from build123d import *

# Parameters (mm, degrees)
BOSS_EXTRUDE1_DEPTH = 11
SKETCH3_W           = 22
SKETCH3_H           = 3
BOSS_EXTRUDE2_DEPTH = 14
BOSS_EXTRUDE3_DEPTH = 5
SKETCH5_R           = 1.75
CUT_EXTRUDE1_DEPTH  = 36.096650541
SKETCH6_W           = 9
SKETCH6_H           = 9
BOSS_EXTRUDE4_DEPTH = 5
SKETCH10_R          = 2.25
CUT_EXTRUDE2_DEPTH  = 34.584744739
FILLET1_R           = 0.75
FILLET2_SIZE        = 10
SKETCH12_W          = 9
SKETCH12_H          = 32.0178
BOSS_EXTRUDE5_DEPTH = 62
CUT_EXTRUDE4_DEPTH  = 9
SKETCH14_R          = 2.5
CUT_EXTRUDE5_DEPTH  = 9.75
SKETCH15_R          = 1.7
CUT_EXTRUDE6_DEPTH  = 5
SKETCH16_R          = 2.5
CUT_EXTRUDE7_DEPTH  = 1.6
FILLET3_R           = 0.5
FILLET4_R           = 0.5
SKETCH17_W          = 3.75
SKETCH17_H          = 32.0178
CUT_EXTRUDE9_DEPTH  = 72.375381621
SKETCH18_W          = 9
SKETCH18_H          = 9
BOSS_EXTRUDE6_DEPTH = 5
CUT_EXTRUDE10_REACH = 71.206
SKETCH19_R          = 2.25
FILLET6_START       = -17
FILLET6_DEPTH       = 11
CUT_EXTRUDE11_REACH = 74.1
SKETCH20_W          = 22
SKETCH20_H          = 25
CUT_EXTRUDE12_DEPTH = 75.22605744
FILLET7_START       = 16
FILLET7_DEPTH       = 5.25


with BuildPart() as part:
    # Sketch1 → Boss-Extrude1 (new, symmetric)
    with BuildSketch(Plane(origin=(0, 0, 0), x_dir=(0, 0, -1), z_dir=(1, 0, 0))):
        Polygon((-13.0089, 0), (13.0089, 0), (13.0089, 8.5), (5.7589, 8.5), (5.7589, 7), (-5.7589, 7), (-5.7589, 8.5), (-13.0089, 8.5), align=None)
    extrude(amount=BOSS_EXTRUDE1_DEPTH, both=True)

    # Sketch3 → Boss-Extrude2 (add)
    with BuildSketch(Plane.XZ):
        with Locations((0, -14.5089)):
            Rectangle(SKETCH3_W, SKETCH3_H)
        with Locations((0, 14.5089)):
            Rectangle(SKETCH3_W, SKETCH3_H)
    extrude(amount=-BOSS_EXTRUDE2_DEPTH)

    # Sketch4 → Boss-Extrude3 (add)
    with BuildSketch(Plane(origin=(11, 0, 0), x_dir=(0, 0, -1), z_dir=(1, 0, 0))):
        Polygon((-8.8, 15.7), (-16.0089, 15.7), (-16.0089, 0), (16.0089, 0), (16.0089, 15.7), align=None)
    extrude(amount=BOSS_EXTRUDE3_DEPTH)

    # Sketch5 → Cut-Extrude1 (cut, through all)
    with BuildSketch(Plane(origin=(16, 0, 0), x_dir=(0, 0, -1), z_dir=(1, 0, 0))):
        with Locations((-10.5, 11)):
            Circle(SKETCH5_R)
        with Locations((10.5, 11)):
            Circle(SKETCH5_R)
    extrude(amount=-CUT_EXTRUDE1_DEPTH, mode=Mode.SUBTRACT)

    # Sketch6 → Boss-Extrude4 (add)
    with BuildSketch(Plane.XZ):
        with Locations((11.5, 20.5089)):
            Rectangle(SKETCH6_W, SKETCH6_H)
    extrude(amount=-BOSS_EXTRUDE4_DEPTH)

    # Sketch10 → Cut-Extrude2 (cut, through all)
    with BuildSketch(Plane.XZ):
        with Locations(Location((11.5, 20.5089, 0), (0, 0, 270))):
            Circle(SKETCH10_R)
    extrude(amount=-CUT_EXTRUDE2_DEPTH, mode=Mode.SUBTRACT)

    # Fillet1
    fillet1_edges = [part.edges().sort_by_distance(p)[0] for p in [
        (0, 8.5, 5.7589),
        (0, 8.5, -5.7589),
        (0, 14, -13.0089),
        (11, 14, -14.5089),
        (11, 11.25, -13.0089),
        (11, 14, 14.5089),
        (11, 11.25, 13.0089),
        (0, 14, 13.0089),
        (11, 15.7, 0),
        (16, 15.7, 0),
        (11.5, 5, 25.0089),
    ]]
    fillet(fillet1_edges, radius=FILLET1_R)

    # Fillet2
    # a fillet whose section is not a circle: 10 mm, written as the material it takes off along each edge
    with BuildSketch(Plane(origin=(-11, -25, 16.0089), x_dir=(0, 0, -1), z_dir=(0, 1, 0))) as fillet2_piece_1:
        with BuildLine():
            add(Edge.make_bspline([(FILLET2_SIZE, 0), (FILLET2_SIZE * 0.831801948466, 0), (FILLET2_SIZE * 0.663603896932, 0), (FILLET2_SIZE * 0.292893218813, -FILLET2_SIZE * 0.0716919198361), (FILLET2_SIZE * 0.0716919198361, -FILLET2_SIZE * 0.292893218813), (0, -FILLET2_SIZE * 0.663603896932), (0, -FILLET2_SIZE * 0.831801948466), (0, -FILLET2_SIZE)], knots=[0, 0, 0, 0, 0, 0, 0.5, 0.5, 1, 1, 1, 1, 1, 1], degree=5))
            Line((0, -FILLET2_SIZE), (0, 0))
            Line((0, 0), (FILLET2_SIZE, 0))
        make_face()
    extrude(amount=64, mode=Mode.SUBTRACT)

    # Sketch12 → Boss-Extrude5 (add)
    with BuildSketch(Plane.XZ):
        with Locations((20.5, 0)):
            Rectangle(SKETCH12_W, SKETCH12_H)
    extrude(amount=-BOSS_EXTRUDE5_DEPTH)

    # Sketch13 → Cut-Extrude4 (cut)
    with BuildSketch(Plane(origin=(25, 0, 0), x_dir=(0, 0, -1), z_dir=(1, 0, 0))):
        Polygon((16.0089, 62), (-16.0089, 62), (16.0089, 53.420856347), align=None)
    extrude(amount=-CUT_EXTRUDE4_DEPTH, mode=Mode.SUBTRACT)

    # Sketch14 → Cut-Extrude5 (cut)
    with BuildSketch(Plane(origin=(25, 0, 0), x_dir=(0, 0, -1), z_dir=(1, 0, 0))):
        with Locations((-10.5, 11)):
            Circle(SKETCH14_R)
        with Locations((10.5, 11)):
            Circle(SKETCH14_R)
    extrude(amount=-CUT_EXTRUDE5_DEPTH, mode=Mode.SUBTRACT)

    # Sketch15 → Cut-Extrude6 (cut)
    with BuildSketch(Plane(origin=(0, 53.844562517, -14.427607043), x_dir=(1, 0, 0), z_dir=(0, 0.9659258262890701, -0.25881904510251424))):
        with Locations(Location((19, -5.362925068, 0), (0, 0, 270))):
            Circle(SKETCH15_R)
        with Locations(Location((19, -25.362925068, 0), (0, 0, 270))):
            Circle(SKETCH15_R)
    extrude(amount=-CUT_EXTRUDE6_DEPTH, mode=Mode.SUBTRACT)

    # Sketch16 → Cut-Extrude7 (cut)
    with BuildSketch(Plane(origin=(0, 53.844562517, -14.427607043), x_dir=(1, 0, 0), z_dir=(0, 0.9659258262890701, -0.25881904510251424))):
        with Locations(Location((19, -5.362925068, 0), (0, 0, 270))):
            Circle(SKETCH16_R)
        with Locations(Location((19, -25.362925068, 0), (0, 0, 270))):
            Circle(SKETCH16_R)
    extrude(amount=-CUT_EXTRUDE7_DEPTH, mode=Mode.SUBTRACT)

    # Fillet3
    fillet3_edges = [part.edges().sort_by_distance(p)[0] for p in [
        (19, 54.58554205, -11.662233782),
        (19, 59.761922952, 7.656282744),
    ]]
    fillet(fillet3_edges, radius=FILLET3_R)

    # Fillet4
    fillet4_edges = [part.edges().sort_by_distance(p)[0] for p in [
        (25, 11, 13),
        (25, 11, -8),
    ]]
    fillet(fillet4_edges, radius=FILLET4_R)

    # Sketch17 → Cut-Extrude9 (cut, through all)
    with BuildSketch(Plane(origin=(0, 62, 0), x_dir=(-1, 0, 0), z_dir=(0, -1, 0))):
        with Locations((-23.125, 0)):
            Rectangle(SKETCH17_W, SKETCH17_H)
    extrude(amount=CUT_EXTRUDE9_DEPTH, mode=Mode.SUBTRACT)

    # Fillet5: read off the stored shape, not the designer's step
    # Fillet5 outline → Fillet5 (revolve, cut)
    with BuildSketch(Plane(origin=(0, 11, -10.5), x_dir=(0, 1, 0), z_dir=(0, 0, -1))):
        with BuildLine():
            ThreePointArc((2.5, 20.75), (2.646446609, 21.103553391), (3, 21.25))
            Line((3, 21.25), (2.5, 21.25))
            Line((2.5, 21.25), (2.5, 20.75))
        make_face()
    revolve(axis=Axis((0, 11, -10.5), (1, 0, 0)), mode=Mode.SUBTRACT)

    # Fillet5 2 outline → Fillet5 2 (revolve, cut)
    with BuildSketch(Plane(origin=(0, 11, 10.5), x_dir=(0, 1, 0), z_dir=(0, 0, -1))):
        with BuildLine():
            ThreePointArc((2.5, 20.75), (2.646446609, 21.103553391), (3, 21.25))
            Line((3, 21.25), (2.5, 21.25))
            Line((2.5, 21.25), (2.5, 20.75))
        make_face()
    revolve(axis=Axis((0, 11, 10.5), (1, 0, 0)), mode=Mode.SUBTRACT)

    # Sketch18 → Boss-Extrude6 (add)
    with BuildSketch(Plane.XZ):
        with Locations((25.75, -11.5089)):
            Rectangle(SKETCH18_W, SKETCH18_H)
    extrude(amount=-BOSS_EXTRUDE6_DEPTH)

    # Sketch19 → Cut-Extrude10 (cut, up to next)
    with BuildSketch(Plane(origin=(0, 5, 0), x_dir=(1, 0, 0), z_dir=(0, 1, 0)), mode=Mode.PRIVATE) as cut_extrude10_sk1:
        with Locations(Location((25.75, 11.5089, 0), (0, 0, 270))):
            Circle(SKETCH19_R)
    cut_extrude10_tool1 = extrude(cut_extrude10_sk1.sketch, amount=-CUT_EXTRUDE10_REACH, mode=Mode.PRIVATE) & part.part
    add(cut_extrude10_tool1.solids().sort_by_distance((25.75, 5, -11.5089))[0], mode=Mode.SUBTRACT)

    # Fillet6: read off the stored shape, not the designer's step
    # Fillet6 outline → Fillet6 (cut)
    with BuildSketch(Plane.XY.offset(FILLET6_START)):
        with BuildLine():
            ThreePointArc((29.5, 5), (30.030330086, 4.780330086), (30.25, 4.25))
            Line((30.25, 4.25), (30.25, 5))
            Line((30.25, 5), (29.5, 5))
        make_face()
    extrude(amount=FILLET6_DEPTH, mode=Mode.SUBTRACT)

    # Sketch20 → Cut-Extrude11 (cut, up to next)
    with BuildSketch(Plane.ZY.offset(-16), mode=Mode.PRIVATE) as cut_extrude11_sk1:
        with Locations((-0.0089, 33.2)):
            Rectangle(SKETCH20_W, SKETCH20_H)
    cut_extrude11_tool1 = extrude(cut_extrude11_sk1.sketch, amount=-CUT_EXTRUDE11_REACH, mode=Mode.PRIVATE) & part.part
    add(cut_extrude11_tool1.solids().sort_by_distance((16, 33.2, -0.0089))[0], mode=Mode.SUBTRACT)

    # Sketch21 → Cut-Extrude12 (cut, through all)
    with BuildSketch(Plane(origin=(21.25, 0, 0), x_dir=(0, 0, -1), z_dir=(1, 0, 0))):
        Polygon((16.0089, 5), (16.0089, 53.420856347), (13.435127939, 54.110496492), align=None)
    extrude(amount=-CUT_EXTRUDE12_DEPTH, mode=Mode.SUBTRACT)

    # Fillet7: read off the stored shape, not the designer's step
    # Fillet7 outline → Fillet7 (add)
    with BuildSketch(Plane.YZ.offset(FILLET7_START)):
        with BuildLine():
            ThreePointArc((27.7, -11.0089), (22.750252532, -8.958647468), (20.7, -4.0089))
            Line((20.7, -4.0089), (20.7, -11.0089))
            Line((20.7, -11.0089), (27.7, -11.0089))
        make_face()
        with BuildLine():
            Line((20.7, 10.9911), (20.7, 3.9911))
            ThreePointArc((20.7, 3.9911), (22.750252532, 8.940847468), (27.7, 10.9911))
            Line((27.7, 10.9911), (20.7, 10.9911))
        make_face()
        with BuildLine():
            ThreePointArc((45.7, -4.0089), (43.649747468, -8.958647468), (38.7, -11.0089))
            Line((38.7, -11.0089), (45.7, -11.0089))
            Line((45.7, -11.0089), (45.7, -4.0089))
        make_face()
        with BuildLine():
            Line((45.7, 10.9911), (38.7, 10.9911))
            ThreePointArc((38.7, 10.9911), (43.649747468, 8.940847468), (45.7, 3.9911))
            Line((45.7, 3.9911), (45.7, 10.9911))
        make_face()
    extrude(amount=FILLET7_DEPTH)


solid = part.part
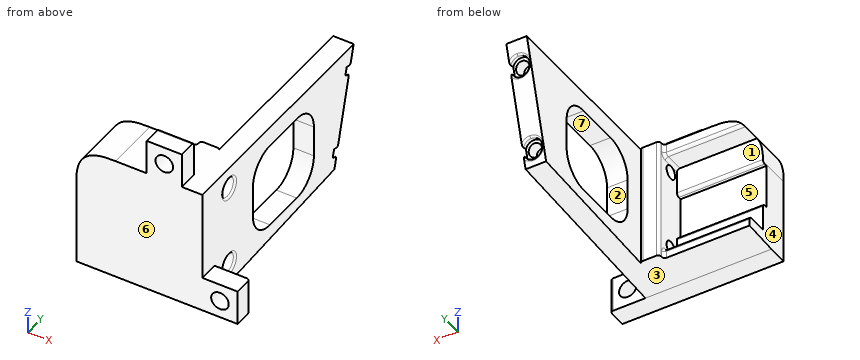
Source: CAD feature listing. Evaluate the final solid. Frame: model axes, mm. Face numbers are marked on the shaded views. A direction names the side the tool comes from. Coordinates: 2 decimals unless noted, no trailing zeros. Loops run counter-clockwise (first coordinate to the right, second up) from the corner with the lowest first, then second, coordinate; pieces in that order, holes last. Notation, with made-up numbers: (86, 23.25) - (130, 23.25) arc R32 cw to (130, 50.25) - close; hole circle Ø3 at (43.25, 10.25). An arc over 180 degrees is marked (long way). One line per item, written item: value. Start each with the question number.
1. Mould query, pull axis Z, two halves, no side actions, for the marked faces 1, 2, 3 and 4. Classes: pulls with the +Z half, pulls with the -Z half, needs draft (parallel to the pull), parting line crosses it, or undercut.
2. Ray query, L1, parallel to Z at x = 17.25, y = 11; L2, parallel to Y at x = -2.5, z = 5; L3, parallel to Y at x = 13, z = -5. Return the intervals inside material, ascending.
3. Contact query for flat-ended pins moving along their axis: P1, Ø1.5, axis at y = 12, z = -10, coming from the +X side; P2, Ø5.5, axis at y = 3.5, z = 21.5, coming from the -X side; P3, Ø6.5, axis at x = 12.5, z = 20, coming from the +Y side. Output: stop coordinate, or through.
4. Section B-B (y = 24.5). Return the cut outline in (x, z).
5. Section A-A (x = 25.75). Return the cut outline in (y, z).
6. Set-up query: the marked faces 5, 6 and 7. Return all of +Z, -Z, +X, -X, +Y, -Y with unobstructed straight access to the full face (end or side cutting, diameter ignored); none if empty.
7. Section C-C (x = 3.5). Return the cut outline in (y, z).
8. Section D-D (y = 11). State how many separate pieces and enclosed holes the cut face has, and give its area (3 significant figures).
Verdict:
1. face 1: undercut
1. face 2: undercut
1. face 3: pulls with the -Z half
1. face 4: needs draft
2. L1: z = -15.69 to -13, -8 to 8, 13 to 16.01
2. L2: y = 0 to 7
2. L3: y = 0 to 15.7
3. P1: stops at x = 15.25
3. P2: stops at x = 7
3. P3: stops at y = 5
4. outline: (16, -14.99) - (21.25, -14.99) - (21.25, -10.23) - (16, -10.23) - close; (16, 10.22) - (21.25, 10.22) - (21.25, 16.01) - (16, 16.01) - close
5. outline: (0, -16.01) - (5, -16.01) - (5, -13.76) - (0, -13.76) - close; (0, -9.26) - (5, -9.26) - (5, -7.01) - (0, -7.01) - close
6. face 5: -X, +Y
6. face 6: +Z, -Z, +X, -X, -Y
6. face 7: +X, -X
7. outline: (0, -16.01) - (5, -16.01) - (14, -15.54) - (14, -13.76) arc R0.75 ccw to (13.25, -13.01) - (8.5, -13.01) - (8.5, -6.51) arc R0.75 ccw to (7.75, -5.76) - (7, -5.76) - (7, 5.76) - (7.75, 5.76) arc R0.75 ccw to (8.5, 6.51) - (8.5, 13.01) - (13.25, 13.01) arc R0.75 ccw to (14, 13.76) - (14, 16.01) - (0, 16.01) - close
8. separate pieces: 3
8. enclosed holes: 0
8. area: 350 mm2
